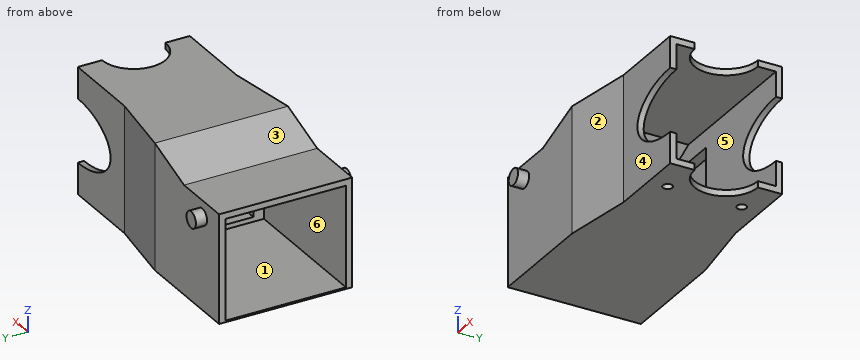
```python
from build123d import *

# Parameters (mm, degrees)
ESQUISSE1_W             = 44.1
ESQUISSE1_H             = 39.27
BOSS_EXTRU_1_DEPTH      = 28.42
ESQUISSE2_W             = 39.7
ESQUISSE2_H             = 34.87
ENL_V_MAT_EXTRU_1_DEPTH = 28.42
ESQUISSE3_R             = 11.1
ENL_V_MAT_EXTRU_2_DEPTH = 50
ESQUISSE4_RX            = 20
ESQUISSE4_RY            = 11.1
ENL_V_MAT_EXTRU_3_DEPTH = 50
ESQUISSE5_R             = 1.65
ENL_V_MAT_EXTRU_4_DEPTH = 10
ESQUISSE6_W             = 64.18
ESQUISSE6_H             = 39.27
BOSS_EXTRU_2_DEPTH      = 2.2
ESQUISSE8_W             = 44.1
ESQUISSE8_H             = 39.27
BOSS_EXTRU_3_DEPTH      = 25
BOSS_EXTRU_4_DEPTH      = 44.1
BOSS_EXTRU_5_START      = -2.2
ESQUISSE13_W            = 39.18
ESQUISSE13_H            = 3.71
BOSS_EXTRU_5_DEPTH      = 2.2
ESQUISSE14_W            = 39.7
ESQUISSE14_H            = 34.87
ENL_V_MAT_EXTRU_5_DEPTH = 25
ESQUISSE17_W            = 38
ESQUISSE17_H            = 46.69
BOSS_EXTRU_6_DEPTH      = 39.18
ESQUISSE18_W            = 35.2475242
ESQUISSE18_H            = 42.29
ENL_V_MAT_EXTRU_6_DEPTH = 50
BOSS_EXTRU_7_DEPTH      = 46.69
CONG_1_R                = 50
ESQUISSE23_R            = 2.85
BOSS_EXTRU_8_DEPTH      = 3.9
BOSS_EXTRU_9_START      = 3.9
ESQUISSE26_R            = 2.85
BOSS_EXTRU_9_DEPTH      = 3.9


with BuildPart() as part:
    # Esquisse1 → Boss.-Extru.1 (new body)
    with BuildSketch(Plane(origin=(0, 0, 0), x_dir=(0, 0, -1), z_dir=(1, 0, 0))):
        Rectangle(ESQUISSE1_W, ESQUISSE1_H)
    extrude(amount=BOSS_EXTRU_1_DEPTH)

    # Esquisse2 → Enlèv. mat.-Extru.1 (cut)
    with BuildSketch(Plane.ZY):
        Rectangle(ESQUISSE2_W, ESQUISSE2_H)
    extrude(amount=-ENL_V_MAT_EXTRU_1_DEPTH, mode=Mode.SUBTRACT)

    # Esquisse3 → Enlèv. mat.-Extru.2 (cut)
    with BuildSketch(Plane.XY.offset(22.05)):
        with Locations((28.42, 0)):
            Circle(ESQUISSE3_R)
    extrude(amount=-ENL_V_MAT_EXTRU_2_DEPTH, mode=Mode.SUBTRACT)

    # Esquisse4 → Enlèv. mat.-Extru.3 (cut)
    with BuildSketch(Plane.XZ.offset(19.635)):
        with Locations(Location((28.42, 0), (0, 0, -180))):
            Ellipse(ESQUISSE4_RX, ESQUISSE4_RY)
    extrude(amount=-ENL_V_MAT_EXTRU_3_DEPTH, mode=Mode.SUBTRACT)

    # Esquisse5 → Enlèv. mat.-Extru.4 (cut)
    with BuildSketch(Plane(origin=(0, 0, -22.05), x_dir=(-1, 0, 0), z_dir=(0, 0, -1))):
        with Locations((-15.27, -12.985)):
            Circle(ESQUISSE5_R)
        with Locations((-15.27, 12.985)):
            Circle(ESQUISSE5_R)
    extrude(amount=-ENL_V_MAT_EXTRU_4_DEPTH, mode=Mode.SUBTRACT)

    # Esquisse6 → Boss.-Extru.2 (add)
    with BuildSketch(Plane(origin=(0, 0, -22.05), x_dir=(-1, 0, 0), z_dir=(0, 0, -1))):
        with Locations((32.09, 0)):
            Rectangle(ESQUISSE6_W, ESQUISSE6_H)
    extrude(amount=-BOSS_EXTRU_2_DEPTH)

    # Esquisse8 → Boss.-Extru.3 (add)
    with BuildSketch(Plane.ZY):
        Rectangle(ESQUISSE8_W, ESQUISSE8_H)
    extrude(amount=BOSS_EXTRU_3_DEPTH)

    # Esquisse10 → Boss.-Extru.4 (add)
    with BuildSketch(Plane.XY.offset(22.05)):
        Polygon((-25, -19.635), (0, -19.635), (-25, -23.345), align=None)
        Polygon((-25, 19.635), (0, 19.635), (-25, 23.345), align=None)
    extrude(amount=-BOSS_EXTRU_4_DEPTH)

    # Esquisse13 → Boss.-Extru.5 (add)
    with BuildSketch(Plane(origin=(0, 0, -22.05), x_dir=(-1, 0, 0), z_dir=(0, 0, -1)).offset(BOSS_EXTRU_5_START)):
        with Locations((44.59, 21.49)):
            Rectangle(ESQUISSE13_W, ESQUISSE13_H)
        with Locations((44.59, -21.49)):
            Rectangle(ESQUISSE13_W, ESQUISSE13_H)
    extrude(amount=BOSS_EXTRU_5_DEPTH)

    # Esquisse14 → Enlèv. mat.-Extru.5 (cut)
    with BuildSketch(Plane(origin=(0, 0, 0), x_dir=(0, 0, -1), z_dir=(1, 0, 0))):
        Rectangle(ESQUISSE14_W, ESQUISSE14_H)
    extrude(amount=-ENL_V_MAT_EXTRU_5_DEPTH, mode=Mode.SUBTRACT)

    # Esquisse17 → Boss.-Extru.6 (add)
    with BuildSketch(Plane.ZY.offset(64.18)):
        with Locations((-3.05, 0)):
            Rectangle(ESQUISSE17_W, ESQUISSE17_H)
    extrude(amount=-BOSS_EXTRU_6_DEPTH)

    # Esquisse18 → Enlèv. mat.-Extru.6 (cut)
    with BuildSketch(Plane.ZY.offset(64.18)):
        with Locations((-3.8737621, 0)):
            Rectangle(ESQUISSE18_W, ESQUISSE18_H)
    extrude(amount=-ENL_V_MAT_EXTRU_6_DEPTH, mode=Mode.SUBTRACT)

    # Esquisse22 → Boss.-Extru.7 (add)
    with BuildSketch(Plane.XZ.offset(23.345)):
        Polygon((-42.845664821, 15.95), (-25, 15.95), (-25, 22.05), align=None)
    extrude(amount=-BOSS_EXTRU_7_DEPTH)

    # Congé1
    # the kernel refuses this fillet: 50 mm, written as the material it takes off along each edge
    with BuildSketch(Plane(origin=(-25, 17.435, 13.75), x_dir=(0, 0, 1), z_dir=(0, -1, 0))) as cong_1_piece_1:
        with BuildLine():
            CenterArc((50, 23.933031567), CONG_1_R, 180, 28.597962222)
            Line((0, 23.933031567), (0, 0))
            Line((0, 0), (6.1, 0))
        make_face()
    extrude(amount=34.87, mode=Mode.SUBTRACT)

    # Esquisse23 → Boss.-Extru.8 (add)
    with BuildSketch(Plane(origin=(0, 23.345, 0), x_dir=(1, 0, 0), z_dir=(0, 1, 0))):
        with Locations(Location((-53.98, -10.3, 0), (0, 0, 180))):
            Circle(ESQUISSE23_R)
    extrude(amount=BOSS_EXTRU_8_DEPTH)

    # Esquisse26 → Boss.-Extru.9 (add)
    with BuildSketch(Plane.XZ.offset(23.345).offset(BOSS_EXTRU_9_START)):
        with Locations(Location((-53.98, 10.3, 0), (0, 0, 180))):
            Circle(ESQUISSE26_R)
    extrude(amount=-BOSS_EXTRU_9_DEPTH)


solid = part.part
```
Work out the finished part from the listing and answer in its coordinate system (mm). Face numbers are marked on the shaded views. A direction names the side the tool comes from. Give positions to 0.01 mm unless a question says otherwise; leave off trailing zeros. Loops run counter-clockwise (first coordinate to the right, second up) from the corner with the lowest first, then second, coordinate; pieces in that order, holes last. Notation, with made-up numbers: M 12.5,-25.75 L 39.5,-25.75 A18 ccw 39.5,-14.75 Z; hole C -12.75,54 d9. An arc over 180 degrees is marked long. One line per item, written item: value. Start each with the question number.
1. Determine the mould class of the marked faces 1, 2 and 3 for opening direction Y: released by +Y, released by -Y, zero draft, split by the parting line, or undercut.
2. Find section D-D (x = 15). State how many separate pieces and enclosed holes the cut face has, and give its area (3 significant figures).
3. Find section C-C (x = -53.98). Give the vertices of the cut face in (y, z) (3 decimals).
4. Find the intervals of material crossed by probe 1 along Y at (x, z) = (15.27, -21) (3 decimals); probe 2 along Y at (x, z) = (15, -21) (3 decimals); probe 3 along Z at (x, y) = (-48.5, 6), in increasing order.
5. Each of these flat-tipped pins is pushed along its axis until it touches: P1, Ø8.5, axis at x = 8.5, z = -7, coming from the -Y side (3 decimals); P2, Ø8, axis at x = -50.5, z = -0.5, coming from the -Y side (3 decimals); P3, Ø10.5, axis at x = -34.5, z = -10.5, coming from the +Y side (3 decimals); P4, Ø12, axis at x = -51, z = 6, coming from the -Y side (3 decimals). Where does it stop, or does it pass through?
6. Find section A-A (y = 0). Give the vertices of the cut face in (x, z).
7. Which of the six approach directions +Z, -Z, +X, -X, +Y, -Y give full straight-line access (tool end or side, diameter ignored) to the marked faces 4, 5 and 6?
8. Find section B-B (z = -12.5). Give the vertices of the cut face in (x, y) (3 decimals).
Reported:
1. face 1: undercut
1. face 2: released by -Y
1. face 3: zero draft
2. separate pieces: 4
2. enclosed holes: 0
2. area: 261 mm²
3. outline: M -27.245,7.45 L -23.345,7.45 L -23.345,-22.05 L 23.345,-22.05 L 23.345,7.45 L 27.245,7.45 L 27.245,13.15 L 23.345,13.15 L 23.345,15.95 L -23.345,15.95 L -23.345,13.15 L -27.245,13.15 Z; hole M -21.145,-21.498 L 21.145,-21.498 L 21.145,13.75 L -21.145,13.75 Z
4. probe 1: y = -19.635 to -14.635, -11.335 to 11.335, 14.635 to 19.635
4. probe 2: y = -19.635 to -14.613, -11.357 to 11.357, 14.613 to 19.635
4. probe 3: z = -22.05 to -21.5, 13.75 to 15.95
5. P1: stops at y = -19.635
5. P2: stops at y = -23.345
5. P3: stops at y = 23.345
5. P4: stops at y = -27.245
6. outline: M -64.18,-22.05 L 17.32,-22.05 L 17.32,-19.85 L -14.18,-19.85 L -14.18,-21.5 L -64.18,-21.5 Z; M -64.18,13.75 L -48.93,13.75 A50 ccw -25,19.85 L 17.32,19.85 L 17.32,22.05 L -25,22.05 L -42.85,15.95 L -64.18,15.95 Z
7. face 4: +Z, -Z, +X, -Y
7. face 5: +X
7. face 6: -X
8. outline: M -64.18,-23.345 L -25,-23.345 L 0,-19.635 L 28.42,-19.635 L 28.42,-17.435 L -14.18,-17.435 L -14.18,-21.145 L -64.18,-21.145 Z; M -64.18,21.145 L -14.18,21.145 L -14.18,17.435 L 28.42,17.435 L 28.42,19.635 L 0,19.635 L -25,23.345 L -64.18,23.345 Z
